For this review, take the finished solid that the model builds, in its own axes (mm). Face numbers are marked on the shaded views. Coordinates: 2 decimals unless noted, no trailing zeros. Loops run counter-clockwise (first coordinate to the right, second up) from the corner with the lowest first, then second, coordinate; pieces in that order, holes last. Notation, with made-up numbers: (43, 5) -> (52, 5) arc R20 ccw to (52, 17) -> close; hole circle Ø8 at (76.25, 47.25). An arc over 180 degrees is marked (long way). Use a Markdown table: item, result.
from build123d import *

# Parameters (mm, degrees)
SKETCH_W        = 117
SKETCH_H        = 70
PAD_DEPTH       = 15
SKETCH001_W     = 113.068136
SKETCH001_H     = 66.343485
POCKET_DEPTH    = 13
SKETCH002_W     = 43.654532
SKETCH002_H     = 15.131113
POCKET001_DEPTH = 2


with BuildPart() as part:
    # Sketch → Pad (new body)
    with BuildSketch(Plane.XY):
        with Locations((-58.5, -35)):
            Rectangle(SKETCH_W, SKETCH_H)
    extrude(amount=PAD_DEPTH)

    # Sketch001 (on Face6 of Pad) → Pocket (cut)
    with BuildSketch(Plane.XY.offset(15)):
        with Locations((-58.329235, -35.028484)):
            Rectangle(SKETCH001_W, SKETCH001_H)
    extrude(amount=-POCKET_DEPTH, mode=Mode.SUBTRACT)

    # Sketch002 (on Face2 of Pocket) → Pocket001 (cut)
    with BuildSketch(Plane.YZ):
        with Locations((-33.794312, 9.565556)):
            Rectangle(SKETCH002_W, SKETCH002_H)
    extrude(amount=-POCKET001_DEPTH, mode=Mode.SUBTRACT)


solid = part.part
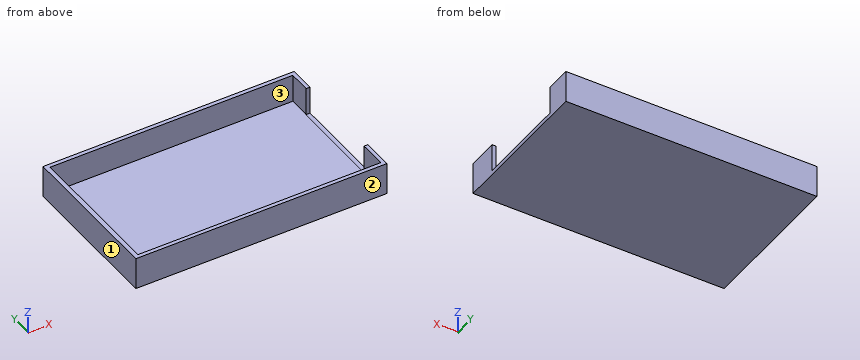
(1) For line 1 along Y through (x, z) = (-5, 8.75); line 2 along X through (y, z) = (-66, 8.75); line 3 along Z through (x, y) = (-21, -49), list the stretches that pass through material, from the lowest coordinate up.
Found:
| item | result |
|---|---|
| line 1 | y = -70 to -68.2, -1.86 to 0 |
| line 2 | x = -117 to -114.86, -1.8 to 0 |
| line 3 | z = 0 to 2 |
(2) Take a section at D-D on y = -59. Write out the cut boundary in (x, z).
Found:
| item | result |
|---|---|
| outline | (-117, 0) -> (0, 0) -> (0, 15) -> (-1.8, 15) -> (-1.8, 2) -> (-114.86, 2) -> (-114.86, 15) -> (-117, 15) -> close |
(3) For pin 1 Ø6 at (x, y) = (-31.5, -61) entering from +Z; pin 2 Ø2 at (y, z) = (-36, 6.5) entering from +X, all flat-tipped, find the tip position at first contact; note any pin that passes through.
Found:
| item | result |
|---|---|
| pin 1 | stops at z = 2 |
| pin 2 | stops at x = -114.86 |
(4) Take a section at A-A on y = -31.5. Write out the cut boundary in (x, z).
Found:
| item | result |
|---|---|
| outline | (-117, 0) -> (0, 0) -> (0, 2) -> (-114.86, 2) -> (-114.86, 15) -> (-117, 15) -> close |
(5) Take a section at C-C on x = -86. Write out the cut boundary in (y, z), plus the area to 3 significant figures.
Found:
| item | result |
|---|---|
| outline | (-70, 0) -> (0, 0) -> (0, 15) -> (-1.86, 15) -> (-1.86, 2) -> (-68.2, 2) -> (-68.2, 15) -> (-70, 15) -> close |
| area | 188 mm^2 |
(6) Mouldability with a two-part tool opening along X and no side actions: class the marked faces 1, 2 and 3 as pulls with the +X half, pulls with the -X half, needs draft (parallel to the pull), parting line crosses it, or undercut.
Found:
| item | result |
|---|---|
| face 1 | pulls with the -X half |
| face 2 | needs draft |
| face 3 | undercut |
(7) Take a section at B-B on z = 7.75. Write out the cut boundary in (x, y).
Found:
| item | result |
|---|---|
| outline | (-117, -70) -> (0, -70) -> (0, -55.62) -> (-1.8, -55.62) -> (-1.8, -68.2) -> (-114.86, -68.2) -> (-114.86, -1.86) -> (-1.8, -1.86) -> (-1.8, -11.97) -> (0, -11.97) -> (0, 0) -> (-117, 0) -> close |
